Print and shaded views of the part. All mm, measured from the part's lowest x, y and z. Give positions to 0.01 mm unless a question says otherwise; leave off trailing zeros. Loops run counter-clockwise (first coordinate to the right, second up) from the corner with the lowest first, then second, coordinate; pieces in that order, holes last. Notation, with made-up numbers: M 53.5,2.5 L 98.5,2.5 A14 cw 98.5,20.5 Z; hole C 62,47 d11. An arc over 180 degrees is marked long. Put each result on its own line as item: value. Start each with the question number.
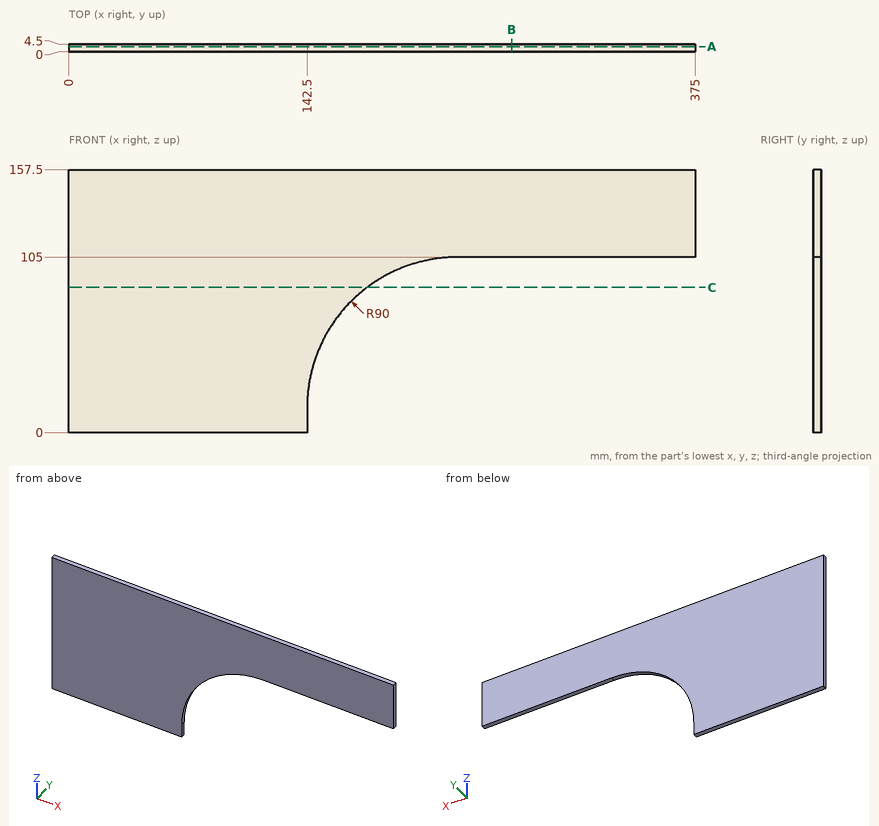
1) Band-saw the part on B-B on x = 265. Give the cut face in (y, z).
2) Wall check: L1, parallel to Z at x = 267.5, y = 4.05; L2, parallel to Z at x = 229.5, y = 1.35; L3, parallel to X at y = 1.4, z = 71.5. Give the ranges that are in metal, low to high.
3) Band-saw the part on A-A on y = 3. Give the cut face in (x, z).
4) Pin check, flat tip, straight feed: pin 1 Ø1.3 at (x, y) = (325, 3) entering from -Z. Stop position of the tip, or through.
5) Band-saw the part on C-C on z = 87. Give the cut face in (x, y).
Evaluation:
1. outline: M 0,105 L 4.5,105 L 4.5,157.5 L 0,157.5 Z
2. L1: 105 to 157.5
2. L2: 104.95 to 157.5
2. L3: 0 to 162.44
3. outline: M 0,0 L 142.5,0 L 142.5,15 A90 cw 232.5,105 L 375,105 L 375,157.5 L 0,157.5 Z
4. pin 1: z = 105
5. outline: M 0,0 L 178.5,0 L 178.5,4.5 L 0,4.5 Z
